Geometry: see drawing. Coordinates: mm, zero at the bounding-box minimum. Round coordinates to 2 decimals unless told otherwise and drop trailing zeros. Order: outer loops, then holes, each group sorted by start corner. A loop starts at its lowest first (then second) coordinate and runs counter-clockwise, first axis right, second up. Notation, with made-up numbers: (49.5, -28) -> (79.5, -28) arc R6 cw to (79.5, -23) -> close; hole circle Ø11 at (8, -19). An arc over 180 degrees is marked (long way). One line per item, written item: value. Start each with the question number.
1) Section A-A (x = 8.8). Return the cut outline in (y, z), and give its area (3 significant figures).
2) Ray query, L1, parallel to Y at x = 1, z = 1.1; L2, parallel to Z at x = 10.75, y = 1; L3, parallel to Y at x = 1, z = 0.15. Return the intervals inside material, ascending.
3) Section C-C (y = 0.7). Return the cut outline in (x, z).
4) Section D-D (y = 6.75). Return the cut outline in (x, z), and give its area (3 significant figures).
5) Section B-B (z = 0.3). Return the cut outline in (x, y).
6) Pin query (flat end, axial travel): P1, Ø2, axis at x = 13, y = 8.5, coming from the -Z side; P2, Ø0.6, axis at y = 6.5, z = 0, coming from the +X side; P3, Ø4, axis at x = 4.5, y = 4, coming from the -Z side; P4, Ø0.6, axis at x = 9.5, z = 0, coming from the +Y side. Return the tip coordinate at first contact, or that it passes through.
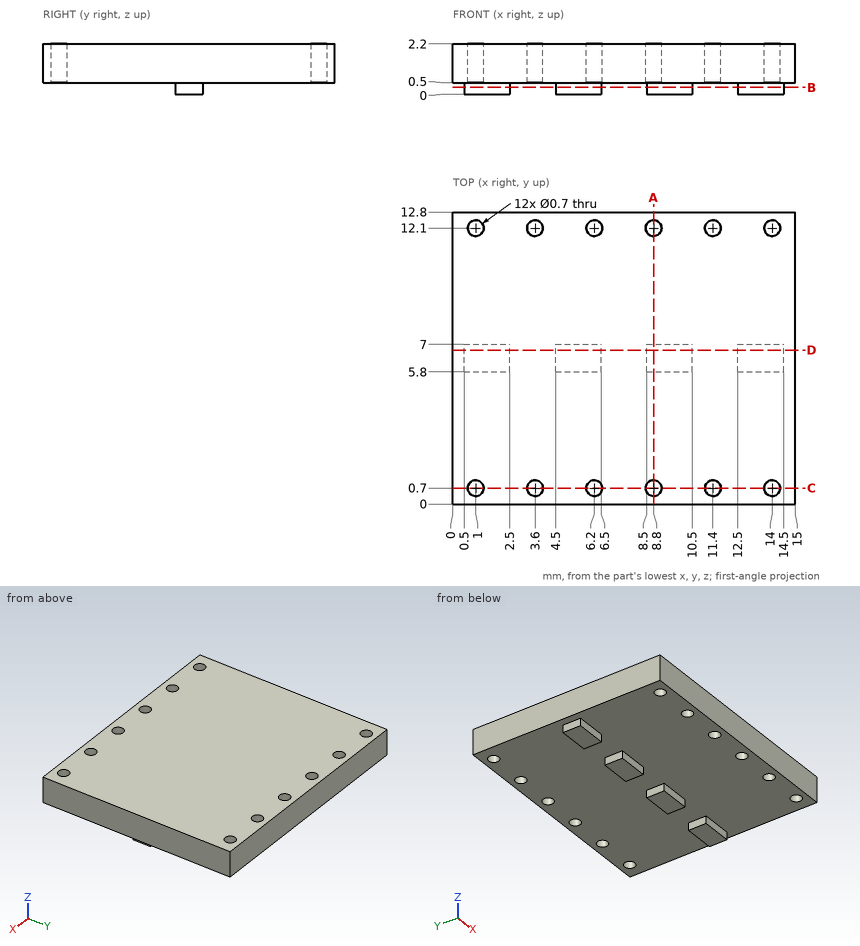
Findings:
1. outline: (0, 0.5) -> (0.35, 0.5) -> (0.35, 2.2) -> (0, 2.2) -> close; (1.05, 0.5) -> (5.8, 0.5) -> (5.8, 0) -> (7, 0) -> (7, 0.5) -> (11.75, 0.5) -> (11.75, 2.2) -> (1.05, 2.2) -> close; (12.45, 0.5) -> (12.8, 0.5) -> (12.8, 2.2) -> (12.45, 2.2) -> close
1. area: 20.0 mm2
2. L1: 0 to 0.35, 1.05 to 11.75, 12.45 to 12.8
2. L2: 0.5 to 2.2
2. L3: 5.8 to 7
3. outline: (0, 0.5) -> (0.65, 0.5) -> (0.65, 2.2) -> (0, 2.2) -> close; (1.35, 0.5) -> (3.25, 0.5) -> (3.25, 2.2) -> (1.35, 2.2) -> close; (3.95, 0.5) -> (5.85, 0.5) -> (5.85, 2.2) -> (3.95, 2.2) -> close; (6.55, 0.5) -> (8.45, 0.5) -> (8.45, 2.2) -> (6.55, 2.2) -> close; (9.15, 0.5) -> (11.05, 0.5) -> (11.05, 2.2) -> (9.15, 2.2) -> close; (11.75, 0.5) -> (13.65, 0.5) -> (13.65, 2.2) -> (11.75, 2.2) -> close; (14.35, 0.5) -> (15, 0.5) -> (15, 2.2) -> (14.35, 2.2) -> close
4. outline: (0, 0.5) -> (0.5, 0.5) -> (0.5, 0) -> (2.5, 0) -> (2.5, 0.5) -> (4.5, 0.5) -> (4.5, 0) -> (6.5, 0) -> (6.5, 0.5) -> (8.5, 0.5) -> (8.5, 0) -> (10.5, 0) -> (10.5, 0.5) -> (12.5, 0.5) -> (12.5, 0) -> (14.5, 0) -> (14.5, 0.5) -> (15, 0.5) -> (15, 2.2) -> (0, 2.2) -> close
4. area: 29.5 mm2
5. outline: (0.5, 5.8) -> (2.5, 5.8) -> (2.5, 7) -> (0.5, 7) -> close; (4.5, 5.8) -> (6.5, 5.8) -> (6.5, 7) -> (4.5, 7) -> close; (8.5, 5.8) -> (10.5, 5.8) -> (10.5, 7) -> (8.5, 7) -> close; (12.5, 5.8) -> (14.5, 5.8) -> (14.5, 7) -> (12.5, 7) -> close
6. P1: z = 0.5
6. P2: x = 14.5
6. P3: z = 0
6. P4: y = 7
